Geometry: final body of the model. Coordinates: model frame, mm. Give positions to 0.01 mm unless a question says otherwise; leave off trailing zeros. Write each loop counter-clockwise with the first axis right and the second up, starting at its lowest first coordinate (ties: lowest second). Pieces come first, ordered by that corner, then holes.
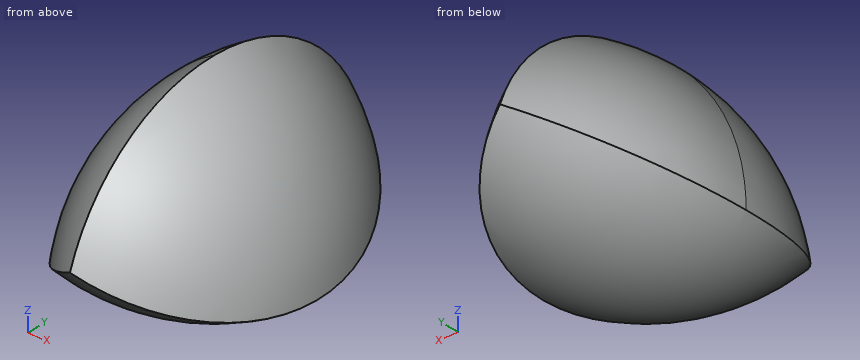
```python
from build123d import *

# Parameters (mm, degrees)
F1_ANGLE_BACK = 90
F1_ANGLE      = 180
F2_ANGLE_BACK = 90
F2_ANGLE      = 180
F3_ANGLE_BACK = 90
F3_ANGLE      = 180


with BuildPart() as f1:
    # F0 (on Front) → F1 (revolve)
    with BuildSketch(Plane.XZ, mode=Mode.PRIVATE) as f1_sk:
        with BuildLine():
            ThreePointArc((10.9985226281, -6.35), (8.0514773719, 4.6485226281), (0, 12.7))
            ThreePointArc((0, 12.7), (-8.0514773719, 4.6485226281), (-10.9985226281, -6.35))
            ThreePointArc((-10.9985226281, -6.35), (0, -9.2970452561), (10.9985226281, -6.35))
        make_face()
    revolve(f1_sk.sketch.rotate(Axis((12.3773198276, 0, -3.961853197), (0.5, 0, 0.8660254038)), -F1_ANGLE_BACK), axis=Axis((12.3773198276, 0, -3.961853197), (0.5, 0, 0.8660254038)), revolution_arc=F1_ANGLE)

    # F0 (on Front) → F2 (revolve, intersect)
    with BuildSketch(Plane.XZ, mode=Mode.PRIVATE) as f2_sk:
        with BuildLine():
            ThreePointArc((10.9985226281, -6.35), (8.0514773719, 4.6485226281), (0, 12.7))
            ThreePointArc((0, 12.7), (-8.0514773719, 4.6485226281), (-10.9985226281, -6.35))
            ThreePointArc((-10.9985226281, -6.35), (0, -9.2970452561), (10.9985226281, -6.35))
        make_face()
    revolve(f2_sk.sketch.rotate(Axis((-2.7575943991, 0, 12.7), (-1, 0, 0)), -F2_ANGLE_BACK), axis=Axis((-2.7575943991, 0, 12.7), (-1, 0, 0)), revolution_arc=F2_ANGLE, mode=Mode.INTERSECT)

    # F0 (on Front) → F3 (revolve, intersect)
    with BuildSketch(Plane.XZ, mode=Mode.PRIVATE) as f3_sk:
        with BuildLine():
            ThreePointArc((10.9985226281, -6.35), (8.0514773719, 4.6485226281), (0, 12.7))
            ThreePointArc((0, 12.7), (-8.0514773719, 4.6485226281), (-10.9985226281, -6.35))
            ThreePointArc((-10.9985226281, -6.35), (0, -9.2970452561), (10.9985226281, -6.35))
        make_face()
    revolve(f3_sk.sketch.rotate(Axis((-9.6197254285, 0, -8.738146803), (0.5, 0, -0.8660254038)), -F3_ANGLE_BACK), axis=Axis((-9.6197254285, 0, -8.738146803), (0.5, 0, -0.8660254038)), revolution_arc=F3_ANGLE, mode=Mode.INTERSECT)


solid = f1.part
```
Item 1: Section C-C, the plane z = 6.5. Return the cut outline in (x, y).
Found:
outline: (0, -14.06) arc R17.85 ccw to (0, 14.06) arc R17.85 ccw to start
Item 2: Pin query (flat end, axial travel): pin 1 Ø4 at (x, y) = (-6.5, 2.5) entering from -Z; pin 2 Ø3 at (x, z) = (0, -6.5) entering from +Y; pin 3 Ø10 at (x, y) = (7.5, -2) entering from +Z. Return the tip coordinate at first contact, or that it passes through.
Found:
pin 1: stops at z = -8.73
pin 2: stops at y = 13.06
pin 3: stops at z = 10.93
Item 3: Line query: L1, parallel to Z at x = -3, y = 15; L2, parallel to X at y = -6.5, z = -3.5; L3, parallel to Y at x = 1, z = -4. Output: solid intervals per line, ascending.
Found:
L1: z = -3.11 to 1.58
L2: x = -9.82 to 9.82
L3: y = -14.28 to 14.28
Item 4: Section B-B, the plane y = 9. Return the cut outline in (x, z), plus the area to 3 significant figures.
Found:
outline: (-9.04, -5.22) arc R20.07 ccw to (9.04, -5.22) arc R20.07 ccw to (0, 10.44) arc R20.07 ccw to start
area: 220 mm2
Item 5: Section A-A, the plane x = -7.75. Return the cut outline in (y, z), plus the area to 3 significant figures.
Found:
outline: (-11.35, -4.47) arc R20.59 ccw to (11.35, -4.47) arc R11.5 ccw to start
area: 218 mm2
Item 6: Section D-D, the plane y = -6. Return the cut outline in (x, z), plus the area to 3 significant figures.
Found:
outline: (-10.16, -5.87) arc R21.16 ccw to (10.16, -5.87) arc R21.16 ccw to (0, 11.73) arc R21.16 ccw to start
area: 286 mm2
